```python
from build123d import *

# Parameters (mm, degrees)
F0_R     = 1.75
F0_R_2   = 11
F0_R_3   = 1.5
F0_R_4   = 2.25
F1_DEPTH = 5
F2_R     = 2.5
F2_R_2   = 1.5
F3_DEPTH = 2.5
F4_SIZE  = 1
F5_SIZE  = 4
F6_R     = 2


with BuildPart() as f1:
    # F0 (on Top) → F1 (new body)
    with BuildSketch(Plane.XY):
        Polygon((12.877052, 25.577868), (-29.122948, 25.577868), (-29.122948, -25.422132), (12.877052, -25.422132), (12.877052, -5.422132), align=None)
        with Locations((-23.622948, -10.922132)):
            Circle(F0_R, mode=Mode.SUBTRACT)
        with Locations((7.377052, -10.922132)):
            Circle(F0_R, mode=Mode.SUBTRACT)
        with Locations((-8.122948, 4.577868)):
            Circle(F0_R_2, mode=Mode.SUBTRACT)
        with Locations((-23.622948, 20.077868)):
            Circle(F0_R, mode=Mode.SUBTRACT)
        with Locations((7.377052, 20.077868)):
            Circle(F0_R, mode=Mode.SUBTRACT)
        Polygon((22.877052, 25.577868), (12.877052, 25.577868), (12.877052, -5.422132), (44.877052, -5.422132), (44.877052, 14.577868), (32.877052, 14.577868), align=None)
        with Locations((39.877052, -0.422132)):
            Circle(F0_R_3, mode=Mode.SUBTRACT)
        with Locations((21.377052, 4.577868)):
            Circle(F0_R_4, mode=Mode.SUBTRACT)
        with Locations((31.377052, 4.577868)):
            Circle(F0_R_4, mode=Mode.SUBTRACT)
        with Locations((39.877052, 9.577868)):
            Circle(F0_R_3, mode=Mode.SUBTRACT)
    extrude(amount=F1_DEPTH)

    # F2 (on face) → F3 (cut)
    with BuildSketch(Plane.XY):
        with Locations((39.890356, -0.446285)):
            Circle(F2_R)
        with Locations((39.877052, -0.422132)):
            Circle(F2_R_2, mode=Mode.SUBTRACT)
        with Locations((39.864622, 9.593817)):
            Circle(F2_R)
    extrude(amount=F3_DEPTH, mode=Mode.SUBTRACT)

    # F4
    f4_edges = [f1.edges().sort_by_distance(p)[0] for p in [
        (-25.372948, 20.077868, 0),
        (5.627052, 20.077868, 0),
        (5.627052, -10.922132, 0),
        (-25.372948, -10.922132, 0),
    ]]
    chamfer(f4_edges, length=F4_SIZE)

    # F5
    f5_edges = [f1.edges().sort_by_distance(p)[0] for p in [
        (-29.122948, 25.577868, 2.5),
        (-29.122948, -25.422132, 2.5),
    ]]
    chamfer(f5_edges, length=F5_SIZE)

    # F6
    f6_edges = [f1.edges().sort_by_distance(p)[0] for p in [
        (44.877052, 14.577868, 2.5),
        (44.877052, -5.422132, 2.5),
    ]]
    fillet(f6_edges, radius=F6_R)


solid = f1.part
```
Source: CAD feature listing. Evaluate the final solid. Frame: model axes, mm. A direction names the side the tool comes from. Give positions to 0.01 mm unless a question says otherwise; leave off trailing zeros. Write each loop counter-clockwise with the first axis right and the second up, starting at its lowest first coordinate (ties: lowest second). Pieces come first, ordered by that corner, then holes.
1. Material intervals for line 1 along X through (y, z) = (-11, 2.85); line 2 along Y through (x, z) = (-17, 4.65); line 3 along X through (y, z) = (11.5, 1.6), sorted ascending.
2. Section query D-D (x = 17.5). Return the cut outline in (y, z).
3. Section query C-C (y = -15). Return the cut outline in (x, z).
4. Section query B-B (x = -18). Return the cut outline in (y, z).
5. Access query for faces 4 (the face through (38, 14.578, 2)), 5 (the face through (7, 0, 0)), 6 (the face through (37.393, -0.336, 1.232)). Directions: +Z, -Z, +X, -X, +Y, -Y. A direction counts if a zero-diameter tool reaches every point of the face in a straight line with its end or side. Return the directions, or none.
6. First-contact query: pin 1 (4 mm diameter, centred on x = 40, y = 9.5, fed in from -Z); pin 2 (1.5 mm diameter, centred on y = -19, z = 1.5, fed in from +X); pin 3 (2.5 mm diameter, centred on x = 24.5, z = 1.5, fed in from -Y). Flat tips, straight axial feed; report the tip coordinate or a pass-through.
7. Pull-direction query (Y, two-part tool) for faces 1 (the face through (28, -5.422, 2)), 2 (the face through (7, 0, 5)), 3 (the face through (8.185, -12.475, 2.972)); classes: +Y half, -Y half, draft (parallel to the pull), parting line (faces both ways), or undercut.
8. Section query A-A (x = -7.5). Return the cut outline in (y, z), then the cut area to 3 significant figures.
Output values:
1. line 1: x = -29.12 to -25.37, -21.87 to 5.63, 9.13 to 12.88
1. line 2: y = -25.42 to -1.92, 11.07 to 25.58
1. line 3: x = -29.12 to -16.67, 0.43 to 38.25, 41.48 to 44.88
2. outline: (-5.42, 0) - (25.58, 0) - (25.58, 5) - (-5.42, 5) - close
3. outline: (-29.12, 0) - (12.88, 0) - (12.88, 5) - (-29.12, 5) - close
4. outline: (-25.42, 0) - (-0.26, 0) - (-0.26, 5) - (-25.42, 5) - close; (9.42, 0) - (25.58, 0) - (25.58, 5) - (9.42, 5) - close
5. face 4: +Z, -Z, +X, +Y
5. face 5: -Z, +X, -X, +Y, -Y
5. face 6: -Z
6. pin 1: stops at z = 2.5
6. pin 2: stops at x = 12.88
6. pin 3: stops at y = -5.42
7. face 1: -Y half
7. face 2: draft
7. face 3: undercut
8. outline: (-25.42, 0) - (-6.4, 0) - (-6.4, 5) - (-25.42, 5) - close; (15.56, 0) - (25.58, 0) - (25.58, 5) - (15.56, 5) - close
8. area: 145 mm2
